Read the model definition and answer for the solid it produces. Units are mm, in the model's axes. Give positions to 0.01 mm unless a question says otherwise; leave off trailing zeros. Order: outer loops, then holes, each group sorted by start corner. A loop starts at its lowest first (then second) coordinate and runs counter-clockwise, first axis right, second up. Notation, with made-up numbers: (75.25, -1) - (112.25, -1) arc R17 cw to (112.25, 28) - close; hole circle Ø11 at (39.25, 74.25). An arc over 180 degrees is marked (long way). Return JSON: item names as keys, results as strings.
```python
from build123d import *

# Parameters (mm, degrees)
SKETCH_1_R      = 1.55
EXTRUDE_1_DEPTH = 1.6


with BuildPart() as part:
    # Эскиз1 → Бобышка-Вытянуть1 (new body)
    with BuildSketch(Plane.XY):
        with BuildLine():
            Line((0, 65), (51, 65))
            Line((51, 65), (51, 55.5))
            ThreePointArc((51, 55.5), (51.292893219, 54.792893219), (52, 54.5))
            Line((52, 54.5), (90, 54.5))
            ThreePointArc((90, 54.5), (90.707106781, 54.792893219), (91, 55.5))
            Line((91, 55.5), (91, 65))
            Line((91, 65), (104, 65))
            Line((104, 65), (104, 0))
            Line((104, 0), (0, 0))
            Line((0, 0), (0, 65))
        make_face()
        with Locations((20.5, 51.5)):
            Circle(SKETCH_1_R, mode=Mode.SUBTRACT)
        with Locations((100.5, 51.5)):
            Circle(SKETCH_1_R, mode=Mode.SUBTRACT)
        with Locations((100.5, 2.5)):
            Circle(SKETCH_1_R, mode=Mode.SUBTRACT)
        with Locations((20.5, 2.5)):
            Circle(SKETCH_1_R, mode=Mode.SUBTRACT)
        with BuildLine():
            Line((62.5, 40.5), (98.5, 40.5))
            ThreePointArc((98.5, 40.5), (99.207106781, 40.207106781), (99.5, 39.5))
            Line((99.5, 39.5), (99.5, 27.5))
            ThreePointArc((99.5, 27.5), (99.207106781, 26.792893219), (98.5, 26.5))
            Line((98.5, 26.5), (62.5, 26.5))
            ThreePointArc((62.5, 26.5), (61.792893219, 26.792893219), (61.5, 27.5))
            Line((61.5, 27.5), (61.5, 39.5))
            ThreePointArc((61.5, 39.5), (61.792893219, 40.207106781), (62.5, 40.5))
        make_face(mode=Mode.SUBTRACT)
    extrude(amount=EXTRUDE_1_DEPTH)


solid = part.part
```
Q1. Consider L1, parallel to Y at x = 100.5, z = 0.9; L2, parallel to Y at x = 67.5, z = 0.6; L3, parallel to Y at x = 94, z = 0.7. Determine where each line is inside the solid, lowest interval first.
Values:
{"L1": "y = 0 to 0.95, 4.05 to 49.95, 53.05 to 65", "L2": "y = 0 to 26.5, 40.5 to 54.5", "L3": "y = 0 to 26.5, 40.5 to 65"}
Q2. A cutting plane is placed at D-D (z = 0.5). Write down the section's boundary in (x, y).
Values:
{"outline": "(0, 0) - (104, 0) - (104, 65) - (91, 65) - (91, 55.5) arc R1 cw to (90, 54.5) - (52, 54.5) arc R1 cw to (51, 55.5) - (51, 65) - (0, 65) - close; hole circle Ø3.1 at (20.5, 2.5); hole circle Ø3.1 at (20.5, 51.5); hole (61.5, 27.5) arc R1 ccw to (62.5, 26.5) - (98.5, 26.5) arc R1 ccw to (99.5, 27.5) - (99.5, 39.5) arc R1 ccw to (98.5, 40.5) - (62.5, 40.5) arc R1 ccw to (61.5, 39.5) - close; hole circle Ø3.1 at (100.5, 2.5); hole circle Ø3.1 at (100.5, 51.5)"}
Q3. A cutting plane is placed at C-C (x = 89). Write down the section's boundary in (y, z).
Values:
{"outline": "(0, 0) - (26.5, 0) - (26.5, 1.6) - (0, 1.6) - close; (40.5, 0) - (54.5, 0) - (54.5, 1.6) - (40.5, 1.6) - close"}
Q4. A cutting plane is placed at A-A (x = 100.5). Write down the section's boundary in (y, z).
Values:
{"outline": "(0, 0) - (0.95, 0) - (0.95, 1.6) - (0, 1.6) - close; (4.05, 0) - (49.95, 0) - (49.95, 1.6) - (4.05, 1.6) - close; (53.05, 0) - (65, 0) - (65, 1.6) - (53.05, 1.6) - close"}
Q5. Determine the mould class of faces 1 (the flat face through (53, 33, 1.6)), 2 (the cylindrical face through (21.932, 1.906, 0.789)), 3 (the cylindrical face through (101.978, 2.966, 0.789)) for opening direction Y: released by +Y, released by -Y, zero draft, split by the parting line, or undercut.
Values:
{"face 1": "zero draft", "face 2": "undercut", "face 3": "undercut"}
Q6. Given pin 1 (0.8 mm diameter, centred on x = 79, z = 0.5, fed in from +Y), flat-ended and moving along its own axis, determine where the tip first touches the part or whether it passes through.
Values:
{"pin 1": "stops at y = 54.5"}
Q7. A cutting plane is placed at B-B (y = 51.5). Write down the section's boundary in (x, z).
Values:
{"outline": "(0, 0) - (18.95, 0) - (18.95, 1.6) - (0, 1.6) - close; (22.05, 0) - (98.95, 0) - (98.95, 1.6) - (22.05, 1.6) - close; (102.05, 0) - (104, 0) - (104, 1.6) - (102.05, 1.6) - close"}
